Design review of the part built by this model. Coordinates are the model's own, in mm. Give positions to 0.01 mm unless a question says otherwise; leave off trailing zeros. Order: outer loops, then holes, each group sorted by start corner. A loop starts at its lowest first (then second) coordinate and runs counter-clockwise, first axis right, second up. Notation, with made-up numbers: M 12.5,-0.5 L 20.5,-0.5 A8 cw 20.5,13.5 Z; hole C -7.75,-2.75 d7. An arc over 180 degrees is marked long. Answer as a JSON object with one key per item and string values.
from build123d import *

# Parameters (mm, degrees)
SKETCH_1_R               = 28
SKETCH_1_R_2             = 2.6
EXTRUDE_1_DEPTH          = 4
CUT_EXTRUDE_2_DEPTH      = 1
CUT_EXTRUDE_2_DEPTH_BACK = 5


with BuildPart() as part:
    # 草图1 → 凸台-拉伸1 (new body)
    with BuildSketch(Plane(origin=(0, 0, 0), x_dir=(1, 0, 0), z_dir=(0, 1, 0))):
        Circle(SKETCH_1_R)
        with Locations((10.5, 18.186533479)):
            Circle(SKETCH_1_R_2, mode=Mode.SUBTRACT)
        with Locations((21, 0)):
            Circle(SKETCH_1_R_2, mode=Mode.SUBTRACT)
        with Locations((10.5, -18.186533479)):
            Circle(SKETCH_1_R_2, mode=Mode.SUBTRACT)
        with Locations((-10.5, -18.186533479)):
            Circle(SKETCH_1_R_2, mode=Mode.SUBTRACT)
        with Locations((-21, 0)):
            Circle(SKETCH_1_R_2, mode=Mode.SUBTRACT)
        with Locations((-10.5, 18.186533479)):
            Circle(SKETCH_1_R_2, mode=Mode.SUBTRACT)
    extrude(amount=EXTRUDE_1_DEPTH)

    # 草图4 → 切除-拉伸2 (cut, two sides)
    with BuildSketch(Plane(origin=(0, 4, 0), x_dir=(1, 0, 0), z_dir=(0, 1, 0))) as cut_extrude_2_sk:
        with BuildLine():
            ThreePointArc((4.758569662, 16.444127766), (7.4999998, 12.990381172), (11.861747108, 12.343105991))
            ThreePointArc((11.861747108, 12.343105991), (17.29701741, 9.986437924), (16.620317219, 4.10102167))
            ThreePointArc((16.620317219, 4.10102167), (15, 2.31e-07), (16.620316904, -4.101021333))
            ThreePointArc((16.620316904, -4.101021333), (17.297017641, -9.986437525), (11.861747557, -12.343106096))
            ThreePointArc((11.861747557, -12.343106096), (7.5000002, -12.990380941), (4.758569796, -16.444127324))
            ThreePointArc((4.758569796, -16.444127324), (2.31e-07, -19.972875449), (-4.758569662, -16.444127766))
            ThreePointArc((-4.758569662, -16.444127766), (-7.4999998, -12.990381172), (-11.861747108, -12.343105991))
            ThreePointArc((-11.861747108, -12.343105991), (-17.29701741, -9.986437924), (-16.620317219, -4.10102167))
            ThreePointArc((-16.620317219, -4.10102167), (-15, -2.31e-07), (-16.620316904, 4.101021333))
            ThreePointArc((-16.620316904, 4.101021333), (-17.297017641, 9.986437525), (-11.861747557, 12.343106096))
            ThreePointArc((-11.861747557, 12.343106096), (-7.5000002, 12.990380941), (-4.758569796, 16.444127324))
            ThreePointArc((-4.758569796, 16.444127324), (-2.31e-07, 19.972875449), (4.758569662, 16.444127766))
        make_face()
    extrude(amount=CUT_EXTRUDE_2_DEPTH, mode=Mode.SUBTRACT)
    extrude(cut_extrude_2_sk.sketch, amount=-CUT_EXTRUDE_2_DEPTH_BACK, mode=Mode.SUBTRACT)


solid = part.part
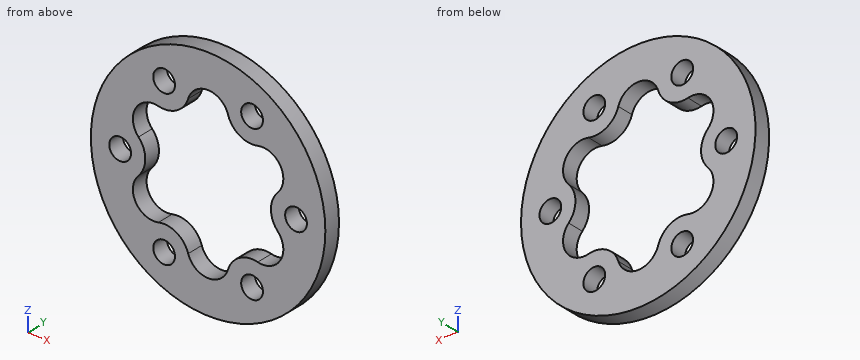
(1) We need section A-A (x = 0). Write out the cut boundary in (y, z).
Checked values:
{"outline": "M 0,-28 L 4,-28 L 4,-19.97 L 0,-19.97 Z; M 0,19.97 L 4,19.97 L 4,28 L 0,28 Z"}
(2) To check wall thickness, follow L1, parallel to X at y = 1.55, z = 0; L2, parallel to Z at x = 10.5, y = 1.4; L3, parallel to Z at x = 12.5, y = 2.5. State the ranges of each line that lie inside material, in increasing order. Write a range as from..to.
Checked values:
{"L1": "x = -28..-23.6, -18.4..-15, 15..18.4, 23.6..28", "L2": "z = -25.96..-20.79, -15.59..-12.19, 12.19..15.59, 20.79..25.96", "L3": "z = -25.05..-19.85, -16.53..-12.45, 12.45..16.53, 19.85..25.05"}
(3) Insertion check: pin 1 (1.5 mm diameter, centred on y = 3.5, z = -10.5, fed in from +X); pin 2 (3 mm diameter, centred on x = 10.5, z = -18.19, fed in from +Y). Each pin has a flat end and moves straight along its axis. Give the tip position at first contact, or say it passes through.
Checked values:
{"pin 1": "stops at x = 26.25", "pin 2": "passes through"}
(4) We need section B-B (z = 0). Write out the cut boundary in (x, y), plus the area to 3 significant figures.
Checked values:
{"outline": "M -28,0 L -23.6,0 L -23.6,4 L -28,4 Z; M -18.4,0 L -15,0 L -15,4 L -18.4,4 Z; M 15,0 L 18.4,0 L 18.4,4 L 15,4 Z; M 23.6,0 L 28,0 L 28,4 L 23.6,4 Z", "area": "62.4 mm^2"}
(5) We need section C-C (x = -10.5). Write out the cut boundary in (y, z), plus the area to 3 significant figures.
Checked values:
{"outline": "M 0,-25.96 L 4,-25.96 L 4,-20.79 L 0,-20.79 Z; M 0,-15.59 L 4,-15.59 L 4,-12.19 L 0,-12.19 Z; M 0,12.19 L 4,12.19 L 4,15.59 L 0,15.59 Z; M 0,20.79 L 4,20.79 L 4,25.96 L 0,25.96 Z", "area": "68.6 mm^2"}
(6) We need section D-D (z = 6.5). Write out the cut boundary in (x, y), plus the area to 3 significant figures.
Checked values:
{"outline": "M -27.24,0 L -17.86,0 L -17.86,4 L -27.24,4 Z; M 17.86,0 L 27.24,0 L 27.24,4 L 17.86,4 Z", "area": "75.0 mm^2"}
